from build123d import *

# Parameters (mm, degrees)
F0_R     = 12.7
F1_DEPTH = 63.5
F3_D     = 12.7
F4_R     = 2.54


with BuildPart() as f1:
    # F0 (on Front) → F1 (new body, symmetric)
    with BuildSketch(Plane.XZ):
        Circle(F0_R)
    extrude(amount=F1_DEPTH, both=True)

    # F3 (through all)
    with Locations(Plane(origin=(0, 63.5, 0), x_dir=(-1, 0, 0), z_dir=(0, 1, 0))):
        with Locations((0, 0)):
            Hole(F3_D / 2)

    # F4
    f4_edges = [f1.edges().sort_by_distance(p)[0] for p in [
        (-12.7, -63.5, 0),
        (-12.7, 63.5, 0),
        (6.35, 63.5, 0),
        (6.35, -63.5, 0),
    ]]
    fillet(f4_edges, radius=F4_R)


solid = f1.part
Source: CAD feature listing. Evaluate the final solid. Frame: model axes, mm. Coordinates: 2 decimals unless noted, no trailing zeros. Loops run counter-clockwise (first coordinate to the right, second up) from the corner with the lowest first, then second, coordinate; pieces in that order, holes last. Notation, with made-up numbers: M 70,52 L 80,52 A27 cw 80,86 Z; hole C -38,9.5 d8. An arc over 180 degrees is marked long. Answer in a Markdown table with one row per item.
Q1. Section C-C on y = -8.5. Return the cut outline in (x, z), plus the area to 3 significant figures.
Answers below:
| item | result |
|---|---|
| outline | C 0,0 d25.4; hole C 0,0 d12.7 |
| area | 380 mm^2 |
Q2. Draft query along Z for faces 1 (the cylindrical face through (-2.75, -0.85, -12.4)), 2 (the flat face through (1, -63.5, -9)), 3 (the cylindrical face through (-1.38, -0.85, -6.2)). Return one class per face: pulls with the +Z half, pulls with the -Z half, needs draft (parallel to the pull), parting line crosses it, or undercut.
Answers below:
| item | result |
|---|---|
| face 1 | parting line crosses it |
| face 2 | needs draft |
| face 3 | undercut |
Q3. Section A-A on z = 0. Return the cut outline in (x, y), plus the area to 3 significant figures.
Answers below:
| item | result |
|---|---|
| outline | M -12.7,-60.96 A2.54 ccw -10.16,-63.5 L -8.89,-63.5 A2.54 ccw -6.35,-60.96 L -6.35,60.96 A2.54 ccw -8.89,63.5 L -10.16,63.5 A2.54 ccw -12.7,60.96 Z; M 6.35,-60.96 A2.54 ccw 8.89,-63.5 L 10.16,-63.5 A2.54 ccw 12.7,-60.96 L 12.7,60.96 A2.54 ccw 10.16,63.5 L 8.89,63.5 A2.54 ccw 6.35,60.96 Z |
| area | 1,600 mm^2 |
Q4. Section B-B on x = 0. Return the cut outline in (y, z).
Answers below:
| item | result |
|---|---|
| outline | M -63.5,-10.16 A2.54 ccw -60.96,-12.7 L 60.96,-12.7 A2.54 ccw 63.5,-10.16 L 63.5,-8.89 A2.54 ccw 60.96,-6.35 L -60.96,-6.35 A2.54 ccw -63.5,-8.89 Z; M -63.5,8.89 A2.54 ccw -60.96,6.35 L 60.96,6.35 A2.54 ccw 63.5,8.89 L 63.5,10.16 A2.54 ccw 60.96,12.7 L -60.96,12.7 A2.54 ccw -63.5,10.16 Z |
Q5. Ray query, probe 1 along Z at (x, y) = (0, 27.5); probe 2 along X at (y, z) = (25, -2.75); probe 3 along Z at (x, y) = (-4, 49). Return the intervals inside material, ascending. Write a range as from..to.
Answers below:
| item | result |
|---|---|
| probe 1 | z = -12.7..-6.35, 6.35..12.7 |
| probe 2 | x = -12.4..-5.72, 5.72..12.4 |
| probe 3 | z = -12.05..-4.93, 4.93..12.05 |
Q6. First-contact query: pin 1 (1 mm diameter, centred on x = 9.5, z = 8, fed in from -Y); pin 2 (4 mm diameter, centred on x = 4.5, z = -1, fed in from -Y); pin 3 (3 mm diameter, centred on x = 7.5, z = 0.5, fed in from -Y); pin 4 (5 mm diameter, centred on x = -10, y = 0.5, fed in from +Z). Flat tips, straight axial feed; report the tip coordinate or a pass-through.
Answers below:
| item | result |
|---|---|
| pin 1 | stops at y = -62.79 |
| pin 2 | stops at y = -62.08 |
| pin 3 | stops at y = -63.5 |
| pin 4 | stops at z = 10.25 |
